```python
from build123d import *

# Parameters (mm, degrees)
F0_R          = 2
F1_DEPTH      = 40
F2_W          = 32
F2_H          = 13
F3_DEPTH      = 38.001
F3_DEPTH_BACK = 25


with BuildPart() as f1:
    # F0 (on Front) → F1 (new body)
    with BuildSketch(Plane.XZ):
        with BuildLine():
            Line((30, 8), (0, 8))
            ThreePointArc((0, 8), (-8, 0), (0, -8))
            Line((0, -8), (30, -8))
            ThreePointArc((30, -8), (38, 0), (30, 8))
        make_face()
        Circle(F0_R, mode=Mode.SUBTRACT)
        with Locations((30, 0)):
            Circle(F0_R, mode=Mode.SUBTRACT)
    extrude(amount=F1_DEPTH)

    # F2 (on Right) → F3 (cut, two sides)
    with BuildSketch(Plane.YZ) as f3_sk:
        with Locations((-20, 1.5)):
            Rectangle(F2_W, F2_H)
    extrude(amount=F3_DEPTH, mode=Mode.SUBTRACT)
    extrude(f3_sk.sketch, amount=-F3_DEPTH_BACK, mode=Mode.SUBTRACT)


solid = f1.part
```
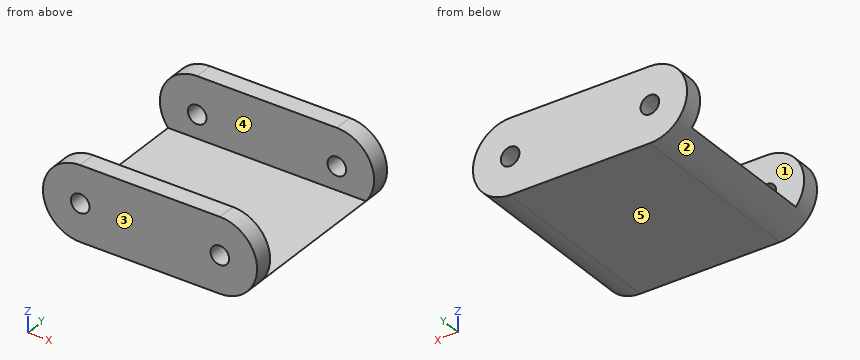
The model under review builds one solid part; all positions refer to its coordinate system, in mm. Face numbers are marked on the shaded views. A direction names the side the tool comes from. Coordinates: 2 decimals unless noted, no trailing zeros. Write each loop counter-clockwise with the first axis right and the second up, starting at its lowest first coordinate (ties: lowest second). Pieces come first, ordered by that corner, then holes. Notation, with made-up numbers: (-14.75, 23) - (-6.75, 23) arc R30 cw to (-6.75, 50) - close; hole circle Ø11 at (39, -10.75). An arc over 180 degrees is marked (long way). Answer in a Markdown table with one row per item. Add a question column.
Q1. To check wall thickness, follow line 1 along X through (y, z) = (-2.8, 0); line 2 along Y through (x, z) = (-3, -3); line 3 along Z through (x, y) = (30, -37). State the ranges of each line that lie inside material, in increasing order. Write a range as from..to.
Q2. Consider section D-D on x = 8. Give the boundary of the cut face in (y, z), then the cut area to 3 significant figures.
Q3. For the marked faces 4 and 5, list the 3-axis set-ups (+Z, -Z, +X, -X, +Y, -Y) from which the entire face can be reached by the end or side of a thin tool; tool diameter is ignored.
Q4. Consider section C-C on z = 4.25. Give the boundary of the cut face in (x, y), then the cut area to 3 significant figures.
Q5. Draft analysis for pull direction Y (two halves, no side actions). For the marked faces 1, 2 and 3, state which applies: +Y half, -Y half, draft (parallel to the pull), parting line (faces both ways), or undercut.
Q6. Clearance check with flat-ended pins moving along their axes: pin 1 (6 mm diameter, centred on y = -9.5, z = 0.5, fed in from -X); pin 2 (6 mm diameter, centred on x = -2, y = -11, fed in from +Z). State where each tip first meets the part, or that it passes through.
Q7. Consider section B-B on x = 31. Give the boundary of the cut face in (y, z).
Q8. Consider section A-A on z = 0. Give the boundary of the cut face in (x, y).
Answers below:
| question | item | result |
|---|---|---|
| 1 | line 1 | -8..-2, 2..28, 32..38 |
| 1 | line 2 | -40..-36, -4..0 |
| 1 | line 3 | -8..-2, 2..8 |
| 2 | outline | (-40, -8) - (0, -8) - (0, 8) - (-4, 8) - (-4, -5) - (-36, -5) - (-36, 8) - (-40, 8) - close |
| 2 | area | 224 mm² |
| 3 | face 4 | +Z, +X, -X |
| 3 | face 5 | -Z, +X, -X, +Y, -Y |
| 4 | outline | (-6.78, -40) - (36.78, -40) - (36.78, -36) - (-6.78, -36) - close; (-6.78, -4) - (36.78, -4) - (36.78, 0) - (-6.78, 0) - close |
| 4 | area | 348 mm² |
| 5 | face 1 | undercut |
| 5 | face 2 | draft |
| 5 | face 3 | -Y half |
| 6 | pin 1 | through |
| 6 | pin 2 | z = -5 |
| 7 | outline | (-40, -7.94) - (0, -7.94) - (0, -1.73) - (-4, -1.73) - (-4, -5) - (-36, -5) - (-36, -1.73) - (-40, -1.73) - close; (-40, 1.73) - (-36, 1.73) - (-36, 7.94) - (-40, 7.94) - close; (-4, 1.73) - (0, 1.73) - (0, 7.94) - (-4, 7.94) - close |
| 8 | outline | (-8, -40) - (-2, -40) - (-2, -36) - (-8, -36) - close; (-8, -4) - (-2, -4) - (-2, 0) - (-8, 0) - close; (2, -40) - (28, -40) - (28, -36) - (2, -36) - close; (2, -4) - (28, -4) - (28, 0) - (2, 0) - close; (32, -40) - (38, -40) - (38, -36) - (32, -36) - close; (32, -4) - (38, -4) - (38, 0) - (32, 0) - close |
